Verification items for the finished model (mm, model axes). A direction names the side the tool comes from. Round coordinates to 2 decimals unless told otherwise and drop trailing zeros. Write each loop counter-clockwise with the first axis right and the second up, starting at its lowest first coordinate (ties: lowest second). Pieces come first, ordered by that corner, then holes. Notation, with made-up numbers: M 36.5,7.25 L 87.5,7.25 A37 ccw 87.5,46.25 Z; hole C -18.5,2.5 d8. An arc over 180 degrees is marked long. One line per item, written item: value. Start each with the question number.
Item 1: Draft check along X on faces 1 (the face through (0.1, 0.4, 5)), 2 (the face through (15, -3, 0)), 3 (the face through (-15, -3, 0)), 4 (the face through (-23.247, -5.979, -0.143)). Enter one of: +X half, -X half, draft (parallel to the pull), parting line (faces both ways), or undercut.
Item 2: Section check C-C, the plane z = 0. State how many separate pieces and enclosed holes the cut face has, then the cut area to 3 significant figures.
Item 3: Thickness scan on probe 1 along Z at (x, y) = (-20, -8.4); probe 2 along X at (y, z) = (-3.25, 1); probe 3 along X at (y, z) = (-6, 1.75). Record the ranges inside material, lowest first. Write a range as from..to.
Item 4: Gauge pin test, flat ends, axial feed: pin 1 (3 mm diameter, centred on x = -15, z = 1, fed in from +Y); pin 2 (3 mm diameter, centred on y = -1.5, z = -2, fed in from -X); pin 3 (2.5 mm diameter, centred on y = -3, z = 1, fed in from +X). Record the tip position at first contact, or that the pin passes through.
Item 5: Section check D-D, the plane z = -4. Record the cut outline in (x, y).
Item 6: Tool access check on faces 5 (the face through (25, -7, 0)), 6 (the face through (16.6, -4.5, 0.1)), 7 (the face through (21.4, -7.5, 1.4)), 8 (the face through (11.9, -0.57, -0.07)). Record the directions out of +Z, -Z, +X, -X, +Y, -Y that give a thin tool (end or side, any length) a straight path to the whole face; none if there is none.
Item 7: Section check B-B, the plane y = -6. Record the cut outline in (x, z).
Item 8: Section check A-A, the plane x = 20. Record the cut outline in (y, z), then the cut area to 3 significant figures.
from build123d import *

# Parameters (mm, degrees)
BOSS_EXTRUDE1_DEPTH            = 5
FILLET1_R                      = 2
FILLET2_R                      = 4
FILLET3_R                      = 2
FILLET4_R                      = 1
CBORE_FOR_M3_SHCS2_D           = 3.4
CBORE_FOR_M3_SHCS2_CBORE_D     = 6.5
CBORE_FOR_M3_SHCS2_CBORE_DEPTH = 3


with BuildPart() as part:
    # Sketch1 → Boss-Extrude1 (new body, symmetric)
    with BuildSketch(Plane.XY):
        Polygon((-15, 2.5), (15, 2.5), (15, -4.5), (25, -4.5), (25, -10), (15, -10), (12.5, -10), (12.5, 0), (-12.5, 0), (-12.5, -10), (-15, -10), (-25, -10), (-25, -4.5), (-15, -4.5), align=None)
    extrude(amount=BOSS_EXTRUDE1_DEPTH, both=True)

    # Fillet1
    fillet1_edges = [part.edges().sort_by_distance(p)[0] for p in [
        (12.5, 0, 0),
        (-12.5, 0, 0),
    ]]
    fillet(fillet1_edges, radius=FILLET1_R)

    # Fillet2
    fillet2_edges = [part.edges().sort_by_distance(p)[0] for p in [
        (-15, 2.5, 0),
        (15, 2.5, 0),
    ]]
    fillet(fillet2_edges, radius=FILLET2_R)

    # Fillet3
    fillet3_edges = [part.edges().sort_by_distance(p)[0] for p in [
        (25, -7.25, -5),
        (-25, -7.25, -5),
        (-25, -7.25, 5),
        (25, -7.25, 5),
    ]]
    fillet(fillet3_edges, radius=FILLET3_R)

    # Fillet4
    fillet4_edges = [part.edges().sort_by_distance(p)[0] for p in [
        (12.5, -10, 0),
        (-12.5, -10, 0),
    ]]
    fillet(fillet4_edges, radius=FILLET4_R)

    # CBORE for M3 SHCS2 (through all)
    with Locations(Plane(origin=(0, -4.5, 0), x_dir=(1, 0, 0), z_dir=(0, 1, 0))):
        with Locations((20, 0), (-20, 0)):
            CounterBoreHole(CBORE_FOR_M3_SHCS2_D / 2, CBORE_FOR_M3_SHCS2_CBORE_D / 2, CBORE_FOR_M3_SHCS2_CBORE_DEPTH)


solid = part.part
Response values:
1. face 1: draft
1. face 2: +X half
1. face 3: -X half
1. face 4: undercut
2. separate pieces: 3
2. enclosed holes: 0
2. area: 173 mm2
3. probe 1: z = -5..-1.7, 1.7..5
3. probe 2: x = -15..-12.5, 12.5..15
3. probe 3: x = -25..-22.74, -17.26..-12.5, 12.5..17.26, 22.74..25
4. pin 1: stops at y = 1.62
4. pin 2: stops at x = -15
4. pin 3: stops at x = 15
5. outline: M -24.73,-10 L -13.5,-10 A1 ccw -12.5,-9 L -12.5,-2 A2 cw -10.5,0 L 10.5,0 A2 cw 12.5,-2 L 12.5,-9 A1 ccw 13.5,-10 L 24.73,-10 L 24.73,-4.5 L 15,-4.5 L 15,-1.5 A4 ccw 11,2.5 L -11,2.5 A4 ccw -15,-1.5 L -15,-4.5 L -24.73,-4.5 Z
6. face 5: +Z, -Z, +X, +Y, -Y
6. face 6: +Z, -Z, +X, +Y
6. face 7: +Y
6. face 8: +Z, -Z, -Y
7. outline: M -25,-3 A2 ccw -23,-5 L -12.5,-5 L -12.5,5 L -23,5 A2 ccw -25,3 Z; M 12.5,-5 L 23,-5 A2 ccw 25,-3 L 25,3 A2 ccw 23,5 L 12.5,5 Z; hole C -20,0 d6.5; hole C 20,0 d6.5
8. outline: M -10,-5 L -4.5,-5 L -4.5,-3.25 L -7.5,-3.25 L -7.5,-1.7 L -10,-1.7 Z; M -10,1.7 L -7.5,1.7 L -7.5,3.25 L -4.5,3.25 L -4.5,5 L -10,5 Z
8. area: 27.0 mm2
